Geometry: final body of the model. Coordinates: model frame, mm. Face numbers are marked on the shaded views. A direction names the side the tool comes from. Round coordinates to 2 decimals unless told otherwise and drop trailing zeros. Write each loop counter-clockwise with the first axis right and the second up, starting at its lowest first coordinate (ties: lowest second). Pieces come first, ordered by that corner, then holes.
from build123d import *

# Parameters (mm, degrees)
F0_W     = 90
F0_H     = 60
F1_DEPTH = 60
F3_DEPTH = 60.001
F5_DEPTH = 60


with BuildPart() as f1:
    # F0 (on Front) → F1 (new body)
    with BuildSketch(Plane.XZ):
        Rectangle(F0_W, F0_H)
    extrude(amount=F1_DEPTH)

    # F2 (on face) → F3 (cut, through all)
    with BuildSketch(Plane.XY.offset(30)):
        with BuildLine():
            Line((45, -52.5), (45, -7.5))
            ThreePointArc((45, -7.5), (22.5, -30), (45, -52.5))
        make_face()
    extrude(amount=-F3_DEPTH, mode=Mode.SUBTRACT)

    # F4 (on face) → F5 (cut)
    with BuildSketch(Plane(origin=(-45, 0, 0), x_dir=(0, -1, 0), z_dir=(-1, 0, 0))):
        with BuildLine():
            Line((0, 30), (0, -10))
            ThreePointArc((0, -10), (28.284271, 1.715729), (40, 30))
            Line((40, 30), (0, 30))
        make_face()
    extrude(amount=-F5_DEPTH, mode=Mode.SUBTRACT)


solid = f1.part
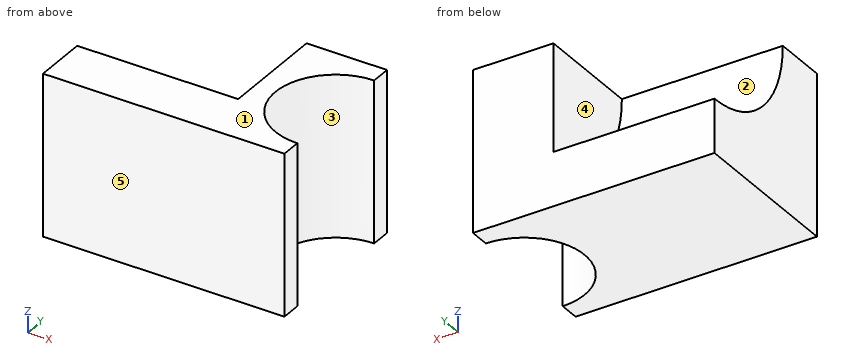
1) First-contact query: P1, Ø1.5, axis at x = -9, y = -10.5, coming from the +Z side; P2, Ø2, axis at y = -44.5, z = -4, coming from the +X side; P3, Ø4, axis at y = -13.5, z = 14, coming from the -X side. Flat tips, straight axial feed; report the tip coordinate or a pass-through.
2) Section C-C on y = -23. Output: boundary loops of the cut face in (x, z), plus the area to 3 significant figures.
3) Draft query along Y for the marked faces 3, 4 and 5. Return one class per face: pulls with the +Y half, pulls with the -Y half, needs draft (parallel to the pull), parting line crosses it, or undercut.
4) Reachability of the marked faces 1 and 2 from +Z, -Z, +X, -X, +Y, -Y: full face, straight path, thin tool, end or side. Return the list, or none.
5) Section B-B on z = 8. Output: boundary loops of the cut face in (x, y).
6) Section A-A on x = -8. Output: boundary loops of the cut face in (y, z), plus the area to 3 significant figures.
7) Line query: probe 1 along X at (y, z) = (-29, 2); probe 2 along X at (y, z) = (-3.5, 18); probe 3 along Y at (x, z) = (37, -8.5). Output: solid intervals per line, ascending.
8) Section D-D on z = -19.5. Output: boundary loops of the cut face in (x, y).
Filled in:
1. P1: stops at z = -8.39
1. P2: stops at x = 28.69
1. P3: stops at x = 15
2. outline: (-45, -30) - (23.62, -30) - (23.62, 30) - (15, 30) - (15, -2.73) - (-45, -2.73) - close
2. area: 2,150 mm2
3. face 3: undercut
3. face 4: needs draft
3. face 5: pulls with the -Y half
4. face 1: +Z, +X, -X, +Y, -Y
4. face 2: +Z, -X, +Y
5. outline: (-45, -60) - (45, -60) - (45, -52.5) arc R22.5 cw to (45, -7.5) - (45, 0) - (15, 0) - (15, -33.41) - (-45, -33.41) - close
6. outline: (-60, -30) - (0, -30) - (0, -10) arc R40 cw to (-40, 30) - (-60, 30) - close
6. area: 2,340 mm2
7. probe 1: x = -45 to 22.52
7. probe 2: x = 15 to 45
7. probe 3: y = -60 to -51.03, -8.97 to 0
8. outline: (-45, -60) - (45, -60) - (45, -52.5) arc R22.5 cw to (45, -7.5) - (45, 0) - (-45, 0) - close
